Here's how the part is built. I have some questions about the finished solid (model axes, mm). Coordinates: 2 decimals unless noted, no trailing zeros. Loops run counter-clockwise (first coordinate to the right, second up) from the corner with the lowest first, then second, coordinate; pieces in that order, holes last. Notation, with made-up numbers: (33, -2) -> (53, -2) arc R25 ccw to (53, 33) -> close; hole circle Ø6 at (9, 24). An arc over 180 degrees is marked (long way). Use CSV: the item, a comma, the result in double quotes. Start each with the question number.
from build123d import *

# Parameters (mm, degrees)
ESBO_O1_W                = 100
ESBO_O1_H                = 40
RESSALTO_EXTRUS_O1_DEPTH = 5
FILETE1_R                = 5
ESBO_O2_R                = 3
CORTE_EXTRUS_O1_DEPTH    = 5


with BuildPart() as part:
    # Esboço1 → Ressalto-extrusão1 (new body)
    with BuildSketch(Plane(origin=(0, 0, 0), x_dir=(1, 0, 0), z_dir=(0, 1, 0))):
        Rectangle(ESBO_O1_W, ESBO_O1_H)
    extrude(amount=RESSALTO_EXTRUS_O1_DEPTH)

    # Filete1
    filete1_edges = [part.edges().sort_by_distance(p)[0] for p in [
        (-50, 2.5, -20),
        (50, 2.5, -20),
        (50, 2.5, 20),
        (-50, 2.5, 20),
    ]]
    fillet(filete1_edges, radius=FILETE1_R)

    # Esboço2 → Corte-extrusão1 (cut)
    with BuildSketch(Plane(origin=(0, 5, 0), x_dir=(1, 0, 0), z_dir=(0, 1, 0))):
        with Locations(Location((-35, 0, 0), (0, 0, 270))):
            Circle(ESBO_O2_R)
        with Locations(Location((35, 0, 0), (0, 0, 270))):
            Circle(ESBO_O2_R)
    extrude(amount=-CORTE_EXTRUS_O1_DEPTH, mode=Mode.SUBTRACT)


solid = part.part
1) Please list where these lines run through material, in increasing order: L1, parallel to X at y = 2.8, z = 0; L2, parallel to X at y = 3, z = 1; L3, parallel to Z at x = 36, y = 2.35. Write a range as [from, to].
2) I want a section at A-A, the plane x = 35. Please give me the cut outline in (y, z), plus the area to 3 significant figures.
3) I want a section at D-D, the plane x = -36. Please give me the cut outline in (y, z).
4) I want a section at C-C, the plane z = 0. Please give me the cut outline in (x, y), plus the area to 3 significant figures.
5) Thinking about a two-plate mould opening in Z: for faces 1 (the face through (37.53, 2.54, 1.61)), 2 (the face through (-1, 2, 20)), 3 (the face through (-1, 2, -20)), which applies, pulls with the +Z half, pulls with the -Z half, needs draft (parallel to the pull), parting line crosses it, or undercut?
6) I want a section at B-B, the plane y = 3. Please give me the cut outline in (x, z), plus the area to 3 significant figures.
Return value:
1,L1,"x = [-50, -38], [-32, 32], [38, 50]"
1,L2,"x = [-50, -37.83], [-32.17, 32.17], [37.83, 50]"
1,L3,"z = [-20, -2.83], [2.83, 20]"
2,outline,"(0, -20) -> (5, -20) -> (5, -3) -> (0, -3) -> close; (0, 3) -> (5, 3) -> (5, 20) -> (0, 20) -> close"
2,area,"170 mm²"
3,outline,"(0, -20) -> (5, -20) -> (5, -2.83) -> (0, -2.83) -> close; (0, 2.83) -> (5, 2.83) -> (5, 20) -> (0, 20) -> close"
4,outline,"(-50, 0) -> (-38, 0) -> (-38, 5) -> (-50, 5) -> close; (-32, 0) -> (32, 0) -> (32, 5) -> (-32, 5) -> close; (38, 0) -> (50, 0) -> (50, 5) -> (38, 5) -> close"
4,area,"440 mm²"
5,face 1,"undercut"
5,face 2,"pulls with the +Z half"
5,face 3,"pulls with the -Z half"
6,outline,"(-50, -15) arc R5 ccw to (-45, -20) -> (45, -20) arc R5 ccw to (50, -15) -> (50, 15) arc R5 ccw to (45, 20) -> (-45, 20) arc R5 ccw to (-50, 15) -> close; hole circle Ø6 at (-35, 0); hole circle Ø6 at (35, 0)"
6,area,"3,920 mm²"
